```python
from build123d import *

# Parameters (mm, degrees)
SKETCH008_W                        = 48
SKETCH008_H                        = 75.5
PAD003_DEPTH                       = 1.6
SKETCH009_W                        = 12.7
SKETCH009_H                        = 12.7
PAD005_DEPTH                       = 1.6
SKETCH010_R                        = 1.25
SKETCH010_R_2                      = 1.5
POCKET005_DEPTH                    = 1.601
SKETCH020_R                        = 0.5
POCKET010_DEPTH                    = 180.6483680343
SKETCH020_LINEARPATTERN002_2_R     = 0.5
POCKET010_LINEARPATTERN002_2_DEPTH = 180.6483680343
LINEARPATTERN003_COUNT             = 5
LINEARPATTERN003_PITCH             = 1.27


with BuildPart() as part:
    # Sketch008 → Pad003 (new body)
    with BuildSketch(Plane.XY):
        with Locations((-3, -17.75)):
            Rectangle(SKETCH008_W, SKETCH008_H)
    extrude(amount=PAD003_DEPTH)

    # Sketch009 (on Face6 of Pad003) → Pad005 (join)
    with BuildSketch(Plane.XY.offset(1.6)):
        with Locations((-3.85, -18.15)):
            Rectangle(SKETCH009_W, SKETCH009_H)
    extrude(amount=PAD005_DEPTH)

    # Sketch010 → Pocket005 (cut, through all)
    with BuildSketch(Plane.XY.offset(1.6)):
        with Locations((-24.25, 17.25)):
            Circle(SKETCH010_R)
        with Locations((18.25, -42.75)):
            Circle(SKETCH010_R)
        with Locations((-22.7, 0.7)):
            Circle(SKETCH010_R_2)
        with Locations((15, -37)):
            Circle(SKETCH010_R_2)
    extrude(amount=-POCKET005_DEPTH, mode=Mode.SUBTRACT)

    # Sketch020 (on Face5 of Pocket005) → Pocket010 (cut, through all)
    with BuildSketch(Plane.XY.offset(1.6)):
        with Locations((-3.27, 12.745)):
            Circle(SKETCH020_R)
    pocket010 = extrude(amount=-POCKET010_DEPTH, mode=Mode.SUBTRACT)

    # Sketch020 LinearPattern002 2 → Pocket010 LinearPattern002 2 (cut, through all)
    with BuildSketch(Plane(origin=(2.54, 0, 1.6), x_dir=(1, 0, 0), z_dir=(0, 0, 1))):
        with Locations((-3.27, 12.745)):
            Circle(SKETCH020_LINEARPATTERN002_2_R)
    pocket010_linearpattern002_2 = extrude(amount=-POCKET010_LINEARPATTERN002_2_DEPTH, mode=Mode.SUBTRACT)

    # LinearPattern003: Pocket010, Pocket010 LinearPattern002 2 ×5
    with Locations(*[(0, -i * LINEARPATTERN003_PITCH, 0) for i in range(1, LINEARPATTERN003_COUNT)]):
        add(pocket010, mode=Mode.SUBTRACT)
        add(pocket010_linearpattern002_2, mode=Mode.SUBTRACT)


solid = part.part
```
Model file for the job. Use its own axes, mm. A direction names the side the tool comes from. Round coordinates to 2 decimals unless told otherwise and drop trailing zeros. Write each loop counter-clockwise with the first axis right and the second up, starting at its lowest first coordinate (ties: lowest second). Pieces come first, ordered by that corner, then holes. Notation, with made-up numbers: M 37,-12.5 L 41,-12.5 A22 cw 41,9.5 Z; hole C -10,-14 d11. An arc over 180 degrees is marked long. Put each result on its own line as item: value.
Item 1: Probe L1, parallel to Y at x = -3.27, z = 0.65 (3 decimals); L2, parallel to Y at x = -3, z = 1.25; L3, parallel to Z at x = -1.5, y = -52. List the from-to ranges inside material, lowest first. Write a range as from..to.
Responses:
L1: -55.5..7.165, 8.165..8.435, 9.435..9.705, 10.705..10.975, 11.975..12.245, 13.245..20
L2: -55.5..7.24, 8.09..8.51, 9.36..9.78, 10.63..11.05, 11.9..12.32, 13.17..20
L3: 0..1.6
Item 2: Cut at A-A (x = 15). List the corners of the cut face in (y, z), and give its area (3 significant figures).
Responses:
outline: M -55.5,0 L -38.5,0 L -38.5,1.6 L -55.5,1.6 Z; M -35.5,0 L 20,0 L 20,1.6 L -35.5,1.6 Z
area: 116 mm²
Item 3: Mould opens along Y. For faces 1 (the flat face through (-4, -24.5, 2)), 2 (the cylindrical face through (13.8, -37.9, 0.8)), 3 (the flat face through (-3, 20, 1)) say: +Y half, -Y half, draft (parallel to the pull), parting line (faces both ways), or undercut.
Responses:
face 1: -Y half
face 2: undercut
face 3: +Y half
Item 4: Cut at B-B (y = -42.75). List the corners of the cut face in (x, z), and give its area (3 significant figures).
Responses:
outline: M -27,0 L 17,0 L 17,1.6 L -27,1.6 Z; M 19.5,0 L 21,0 L 21,1.6 L 19.5,1.6 Z
area: 72.8 mm²
Item 5: Flat gauge pins, fed straight in: P1, Ø1.3, axis at x = -6, z = 2.5, coming from the -Y side; P2, Ø1.3, axis at y = -15, z = 2.5, coming from the +X side; P3, Ø0.8, axis at y = -19, z = 2.5, coming from the -X side; P4, Ø2.5, axis at x = -22.7, y = 0.7, coming from the +Z side. Where does each tip first touch, or does it go through?
Responses:
P1: y = -24.5
P2: x = 2.5
P3: x = -10.2
P4: through
Item 6: Tool access for faces 4 (the flat face through (2.5, -18, 2)), 5 (the flat face through (-10.2, -18, 2)), 6 (the flat face through (-3, -17, 0)), 7 (the flat face through (-4, -11.8, 2)): list every direction of +Z, -Z, +X, -X, +Y, -Y with a clear straight run to the whole face (end or side of a thin tool).
Responses:
face 4: +Z, +X, +Y, -Y
face 5: +Z, -X, +Y, -Y
face 6: -Z, +X, -X, +Y, -Y
face 7: +Z, +X, -X, +Y
Item 7: Cut at D-D (z = 2.4). List the corners of the cut face in (x, y), and give its area (3 significant figures).
Responses:
outline: M -10.2,-24.5 L 2.5,-24.5 L 2.5,-11.8 L -10.2,-11.8 Z
area: 161 mm²
Item 8: Cut at C-C (x = -6). List the corners of the cut face in (y, z).
Responses:
outline: M -55.5,0 L 20,0 L 20,1.6 L -11.8,1.6 L -11.8,3.2 L -24.5,3.2 L -24.5,1.6 L -55.5,1.6 Z
